Geometry: see drawing. Coordinates: mm, zero at the bounding-box minimum. Coordinates: 2 decimals unless noted, no trailing zeros. Write each loop counter-clockwise with the first axis right and the second up, starting at its lowest first coordinate (ties: lowest second). Pieces come first, ordered by that corner, then holes. Notation, with made-up numbers: (-40, -10) - (-30, -10) arc R22 cw to (-30, 0) - close; hole circle Ø7 at (24, -21.5). An arc over 180 degrees is marked (long way). One line per question, with ' | ' between items. Start each with the question number.
Q1. Cut plane C-C, the plane z = 7. Return loops of the section in (x, y).
Q2. Cut plane A-A, the plane x = 21. Return loops of the section in (y, z).
Q3. Draft query along X for the marked faces 1 and 2. Return one class per face: +X half, -X half, draft (parallel to the pull), parting line (faces both ways), or undercut.
Q4. Line query: line 1 (Y direction, x = 21, z = 11); line 2 (X direction, y = 39, z = 29.5); line 3 (Y direction, x = 24, z = 26). Output: solid intervals per line, ascending.
Q5. Contact query for flat-ended pins moving along their axis: P1, Ø2, axis at x = 33, z = 15.5, coming from the -Y side; P2, Ø12, axis at x = 35.5, z = 12, coming from the +Y side; P3, Ø5, axis at x = 33.5, y = 31.5, coming from the +Z side; P4, Ø2, axis at y = 18.5, z = 15, coming from the -X side. Output: stop coordinate, or through.
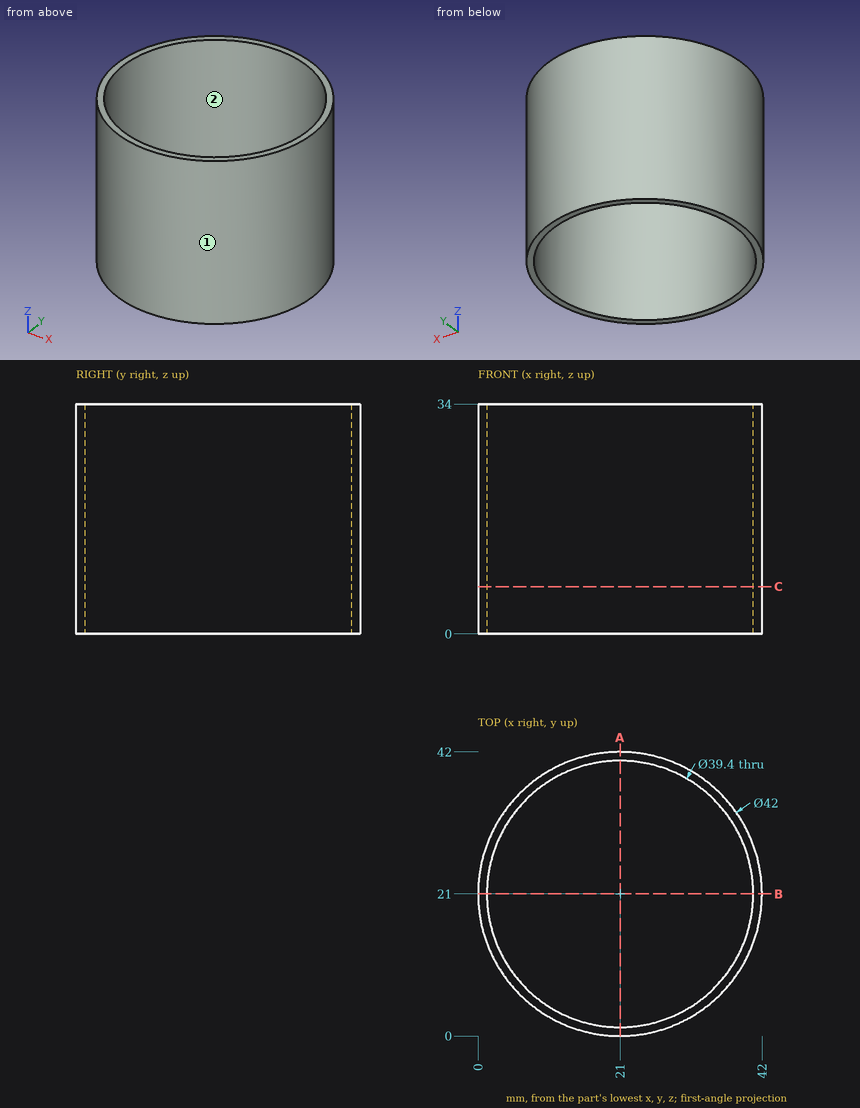
Reply:
1) outline: circle Ø42 at (21, 21); hole circle Ø39.4 at (21, 21)
2) outline: (0, 0) - (1.3, 0) - (1.3, 34) - (0, 34) - close; (40.7, 0) - (42, 0) - (42, 34) - (40.7, 34) - close
3) face 1: parting line | face 2: undercut
4) line 1: y = 0 to 1.3, 40.7 to 42 | line 2: x = 10.18 to 12.99, 29.01 to 31.82 | line 3: y = 0.22 to 1.53, 40.47 to 41.78
5) P1: stops at y = 3.11 | P2: stops at y = 40.2 | P3: passes through | P4: stops at x = 0.05
